from build123d import *

# Parameters (mm, degrees)
BOSS_EXTRUDE1_DEPTH = 183
CUT_EXTRUDE1_REACH  = 188.468


with BuildPart() as part:
    # Sketch1 → Boss-Extrude1 (new body)
    with BuildSketch(Plane.XY):
        with BuildLine():
            Line((0, -2.722861027), (2.5, -2.722861027))
            ThreePointArc((2.5, -2.722861027), (3.914213562, -3.308647465), (4.5, -4.722861027))
            Line((4.5, -4.722861027), (4.5, -7.222861027))
            ThreePointArc((4.5, -7.222861027), (5.378679656, -9.344181371), (7.5, -10.222861027))
            Line((7.5, -10.222861027), (17.5, -10.222861027))
            Line((17.5, -10.222861027), (27.5, -10.222861027))
            ThreePointArc((27.5, -10.222861027), (29.621320344, -9.344181371), (30.5, -7.222861027))
            Line((30.5, -7.222861027), (30.5, -4.722861027))
            ThreePointArc((30.5, -4.722861027), (31.085786438, -3.308647465), (32.5, -2.722861027))
            Line((32.5, -2.722861027), (35, -2.722861027))
            Line((35, -2.722861027), (35, -1.722861027))
            Line((35, -1.722861027), (32.5, -1.722861027))
            ThreePointArc((32.5, -1.722861027), (30.378679656, -2.601540684), (29.5, -4.722861027))
            Line((29.5, -4.722861027), (29.5, -7.222861027))
            ThreePointArc((29.5, -7.222861027), (28.914213562, -8.63707459), (27.5, -9.222861027))
            Line((27.5, -9.222861027), (17.5, -9.222861027))
            Line((17.5, -9.222861027), (7.5, -9.222861027))
            ThreePointArc((7.5, -9.222861027), (6.085786438, -8.63707459), (5.5, -7.222861027))
            Line((5.5, -7.222861027), (5.5, -4.722861027))
            ThreePointArc((5.5, -4.722861027), (4.621320344, -2.601540684), (2.5, -1.722861027))
            Line((2.5, -1.722861027), (0, -1.722861027))
            Line((0, -1.722861027), (0, -2.722861027))
        make_face()
    extrude(amount=BOSS_EXTRUDE1_DEPTH)

    # Sketch2 → Cut-Extrude1 (cut, up to next)
    with BuildSketch(Plane(origin=(0, -9.222861027, 0), x_dir=(1, 0, 0), z_dir=(0, 1, 0)), mode=Mode.PRIVATE) as cut_extrude1_sk1:
        with BuildLine():
            Line((15.5, -178), (15.5, -5))
            ThreePointArc((15.5, -5), (17.5, -3), (19.5, -5))
            Line((19.5, -5), (19.5, -178))
            ThreePointArc((19.5, -178), (17.5, -180), (15.5, -178))
        make_face()
    cut_extrude1_tool1 = extrude(cut_extrude1_sk1.sketch, amount=-CUT_EXTRUDE1_REACH, mode=Mode.PRIVATE) & part.part
    add(cut_extrude1_tool1.solids().sort_by_distance((17.5, -9.222861, 91.5))[0], mode=Mode.SUBTRACT)


solid = part.part
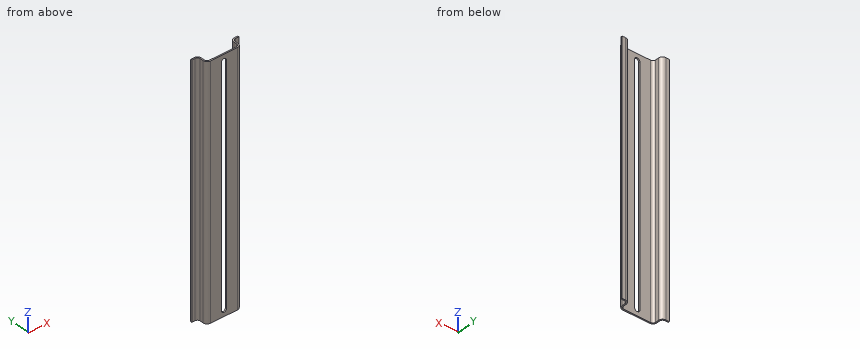
Build history of the part. All positions in model axes, mm. Round coordinates to 2 decimals unless told otherwise and drop trailing zeros. Write each loop counter-clockwise with the first axis right and the second up, starting at its lowest first coordinate (ties: lowest second). Pieces come first, ordered by that corner, then holes. Notation, with made-up numbers: M -26.5,-29.75 L 21.5,-29.75 A35 ccw 21.5,6.25 Z; hole C 64.25,75.25 d11. An arc over 180 degrees is marked long. Answer in a Markdown table with one row per item.
1. Saw through at A-A (x = 17.5). List the corners of the cut face in (y, z), and give its area (3 significant figures).
Geometry check:
| item | result |
|---|---|
| outline | M -10.22,0 L -9.22,0 L -9.22,3 L -10.22,3 Z; M -10.22,180 L -9.22,180 L -9.22,183 L -10.22,183 Z |
| area | 6.00 mm2 |
2. Saw through at B-B (z = 66). List the corners of the cut face in (x, y), and give its area (3 significant figures).
Geometry check:
| item | result |
|---|---|
| outline | M 0,-2.72 L 2.5,-2.72 A2 cw 4.5,-4.72 L 4.5,-7.22 A3 ccw 7.5,-10.22 L 15.5,-10.22 L 15.5,-9.22 L 7.5,-9.22 A2 cw 5.5,-7.22 L 5.5,-4.72 A3 ccw 2.5,-1.72 L 0,-1.72 Z; M 19.5,-10.22 L 27.5,-10.22 A3 ccw 30.5,-7.22 L 30.5,-4.72 A2 cw 32.5,-2.72 L 35,-2.72 L 35,-1.72 L 32.5,-1.72 A3 ccw 29.5,-4.72 L 29.5,-7.22 A2 cw 27.5,-9.22 L 19.5,-9.22 Z |
| area | 41.7 mm2 |
3. Probe L1, parallel to X at y = -6.75, z = 115.5; L2, parallel to X at y = -2.5, z = 116; L3, parallel to Y at x = 25, z = 137. List the from-to ranges inside material, lowest first. Write a range as [from, to].
Geometry check:
| item | result |
|---|---|
| L1 | [4.5, 5.5], [29.5, 30.5] |
| L2 | [0, 4.51], [30.49, 35] |
| L3 | [-10.22, -9.22] |
4. Flat gauge pins, fed straight in: P1, Ø0.8, axis at y = -9.5, z = 89, coming from the +X side; P2, Ø3, axis at x = 33.5, z = 61.5, coming from the -Y side; P3, Ø0.8, axis at y = -5.5, z = 49, coming from the -X side. Where does each tip first touch, or does it go through?
Geometry check:
| item | result |
|---|---|
| P1 | x = 29.84 |
| P2 | y = -2.79 |
| P3 | x = 4.5 |
